from build123d import *

# Parameters (mm, degrees)
BOSS_EXTRUDE1_DEPTH      = 38.1
BOSS_EXTRUDE1_DEPTH_BACK = 38.1
SKETCH1_W                = 76.2
SKETCH1_H                = 76.2
SKETCH1_R                = 4.7625
CHAMFER1_SIZE            = 9.525


with BuildPart() as part:
    # Sketch1 → Boss-Extrude1 (new, two sides: drawn at the far end of the back side and taken through both)
    with BuildSketch(Plane.XY.offset(-BOSS_EXTRUDE1_DEPTH_BACK)):
        with Locations((-6.35, -16.348197115)):
            Rectangle(SKETCH1_W, SKETCH1_H)
        with Locations((-31.75, -35.398197115)):
            Circle(SKETCH1_R, mode=Mode.SUBTRACT)
        with Locations((19.05, -35.398197115)):
            Circle(SKETCH1_R, mode=Mode.SUBTRACT)
    extrude(amount=BOSS_EXTRUDE1_DEPTH + BOSS_EXTRUDE1_DEPTH_BACK)

    # Chamfer1
    chamfer1_edges = [part.edges().sort_by_distance(p)[0] for p in [
        (-6.35, -54.448197115, -38.1),
        (-6.35, 21.751802885, 38.1),
        (-6.35, -54.448197115, 38.1),
        (31.75, -54.448197115, 0),
        (-44.45, -54.448197115, 0),
        (-44.45, 21.751802885, 0),
        (31.75, 21.751802885, 0),
        (-6.35, 21.751802885, -38.1),
    ]]
    chamfer(chamfer1_edges, length=CHAMFER1_SIZE)


solid = part.part
Build history of the part. All positions in model axes, mm. Round coordinates to 2 decimals unless told otherwise and drop trailing zeros. Loops run counter-clockwise (first coordinate to the right, second up) from the corner with the lowest first, then second, coordinate; pieces in that order, holes last. Notation, with made-up numbers: (-10.75, 3) -> (33.25, 3) arc R19 ccw to (33.25, 18) -> close; hole circle Ø10 at (42.25, 31). An arc over 180 degrees is marked (long way). One line per item, written item: value. Start each with the question number.
Q1. Cut at C-C on z = 30. Count the separate pieces of the cut face and the enclosed holes in it, plus the area to 3 significant figures.
Q2. Cut at A-A on x = -31.75. List the corners of the cut face in (y, z) (3 decimals).
Q3. Two-plate mould, pull along X, no slides. Class faces 1 (the face through (-39.621, 17.056, -0.533)), 2 (the face through (-29.55, -39.62, -0.53)), 3 (the face through (-7, -54.448, 0)): released by +X, released by -X, zero draft, split by the parting line, or undercut.
Q4. Cut at B-B on x = -11. List the corners of the cut face in (y, z) (3 decimals), plus the area to 4 significant figures.
Q5. Probe line 1 along X through (y, z) = (-35.5, -29.5); line 2 along Y through (x, z) = (19.05, 1); line 3 along X through (y, z) = (-31, -5.5). List the from-to ranges inside material, lowest first.
Computed:
1. separate pieces: 1
1. enclosed holes: 2
1. area: 5,320 mm²
2. outline: (-54.448, -28.575) -> (-44.923, -38.1) -> (-40.161, -38.1) -> (-40.161, 38.1) -> (-44.923, 38.1) -> (-54.448, 28.575) -> close; (-30.636, -38.1) -> (12.227, -38.1) -> (21.752, -28.575) -> (21.752, 28.575) -> (12.227, 38.1) -> (-30.636, 38.1) -> close
3. face 1: released by -X
3. face 2: undercut
3. face 3: zero draft
4. outline: (-54.448, -28.575) -> (-44.923, -38.1) -> (12.227, -38.1) -> (21.752, -28.575) -> (21.752, 28.575) -> (12.227, 38.1) -> (-44.923, 38.1) -> (-54.448, 28.575) -> close
4. area: 5,625 mm²
5. line 1: -44.45 to -36.51, -26.99 to 14.29, 23.81 to 31.75
5. line 2: -54.45 to -40.16, -30.64 to 21.75
5. line 3: -44.45 to -33.58, -29.92 to 17.22, 20.88 to 31.75
